Work out the finished part from the listing and answer in its coordinate system (mm). Give positions to 0.01 mm unless a question says otherwise; leave off trailing zeros. Loops run counter-clockwise (first coordinate to the right, second up) from the corner with the lowest first, then second, coordinate; pieces in that order, holes last.
```python
from build123d import *

# Parameters (mm, degrees)
SKETCH1_W           = 60
SKETCH1_H           = 38
SKETCH1_R           = 8
SKETCH1_W_2         = 10
SKETCH1_H_2         = 3
SKETCH1_W_3         = 3
SKETCH1_H_3         = 10
BOSS_EXTRUDE1_DEPTH = 3


with BuildPart() as part:
    # Sketch1 → Boss-Extrude1 (new body)
    # profile 1 of 3: a face of its own
    with BuildSketch(Plane.XY):
        with Locations((-2.850678733, -3.932126697)):
            Rectangle(SKETCH1_W, SKETCH1_H)
        with Locations((-16.050678733, -1.932126697)):
            Circle(SKETCH1_R, mode=Mode.SUBTRACT)
        with Locations((10.349321267, -1.932126697)):
            Circle(SKETCH1_R, mode=Mode.SUBTRACT)
        with Locations((-2.850678733, -18.432126697)):
            Rectangle(SKETCH1_W_2, SKETCH1_H_2, mode=Mode.SUBTRACT)
        with Locations((17.149321267, -18.432126697)):
            Rectangle(SKETCH1_W_2, SKETCH1_H_2, mode=Mode.SUBTRACT)
        with Locations((-22.850678733, -18.432126697)):
            Rectangle(SKETCH1_W_2, SKETCH1_H_2, mode=Mode.SUBTRACT)
    # profile 2 of 3: a face of its own
    with BuildSketch(Plane.XY):
        with Locations((-34.350678733, -0.932126697)):
            Rectangle(SKETCH1_W_3, SKETCH1_H_3)
    # profile 3 of 3: a face of its own
    with BuildSketch(Plane.XY):
        with Locations((28.649321267, -0.932126697)):
            Rectangle(SKETCH1_W_3, SKETCH1_H_3)
    extrude(amount=BOSS_EXTRUDE1_DEPTH)


solid = part.part
```
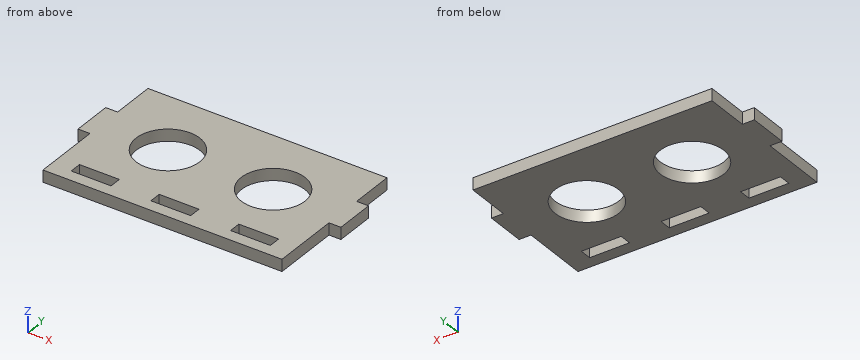
Q1. Section C-C on z = 1.95 is taken. Give the vertices of the cut face in (x, y), plus the area to 3 significant figures.
Q2. Section A-A on x = 20.5 is taken. Give the vertices of the cut face in (y, z).
Q3. Section D-D on y = 2 is taken. Give the vertices of the cut face in (x, z), plus the area to 3 significant figures.
Q4. Section B-B on y = -3.5 is taken. Give the vertices of the cut face in (x, z), plus the area to 3 significant figures.
Q5. Consider line 1 along Y through (x, z) = (-2, 0.8); line 2 along Y through (x, z) = (-21.5, 0.3); line 3 along X through (y, z) = (4.5, 2.2). Determine where each line is inside the solid, lowest interval first.
Q6. Given pin 1 (18.5 mm diameter, centred on x = 10.35, y = -1.93, fed in from +Z); pin 2 (1.5 mm diameter, centred on x = 28, z = 1.5, fed in from -Y); pin 3 (0.9 mm diameter, centred on y = -18.5, z = 1.5, fed in from -X); pin 4 (1.5 mm diameter, centred on x = -35, z = 2, fed in from +Y), each flat-ended and moving along its own axis, determine where each tip first touches the part or whether it passes through.
Check result:
1. outline: (-35.85, -5.93) - (-32.85, -5.93) - (-32.85, -22.93) - (27.15, -22.93) - (27.15, -5.93) - (30.15, -5.93) - (30.15, 4.07) - (27.15, 4.07) - (27.15, 15.07) - (-32.85, 15.07) - (-32.85, 4.07) - (-35.85, 4.07) - close; hole (-27.85, -19.93) - (-17.85, -19.93) - (-17.85, -16.93) - (-27.85, -16.93) - close; hole circle Ø16 at (-16.05, -1.93); hole (-7.85, -19.93) - (2.15, -19.93) - (2.15, -16.93) - (-7.85, -16.93) - close; hole circle Ø16 at (10.35, -1.93); hole (12.15, -19.93) - (22.15, -19.93) - (22.15, -16.93) - (12.15, -16.93) - close
1. area: 1,850 mm2
2. outline: (-22.93, 0) - (-19.93, 0) - (-19.93, 3) - (-22.93, 3) - close; (-16.93, 0) - (15.07, 0) - (15.07, 3) - (-16.93, 3) - close
3. outline: (-35.85, 0) - (-23.02, 0) - (-23.02, 3) - (-35.85, 3) - close; (-9.08, 0) - (3.38, 0) - (3.38, 3) - (-9.08, 3) - close; (17.32, 0) - (30.15, 0) - (30.15, 3) - (17.32, 3) - close
3. area: 114 mm2
4. outline: (-35.85, 0) - (-23.9, 0) - (-23.9, 3) - (-35.85, 3) - close; (-8.21, 0) - (2.5, 0) - (2.5, 3) - (-8.21, 3) - close; (18.19, 0) - (30.15, 0) - (30.15, 3) - (18.19, 3) - close
4. area: 104 mm2
5. line 1: y = -22.93 to -19.93, -16.93 to 15.07
5. line 2: y = -22.93 to -19.93, -16.93 to -7.79, 3.92 to 15.07
5. line 3: x = -32.85 to -20.81, -11.29 to 5.59, 15.11 to 27.15
6. pin 1: stops at z = 3
6. pin 2: stops at y = -5.93
6. pin 3: stops at x = -32.85
6. pin 4: stops at y = 4.07
